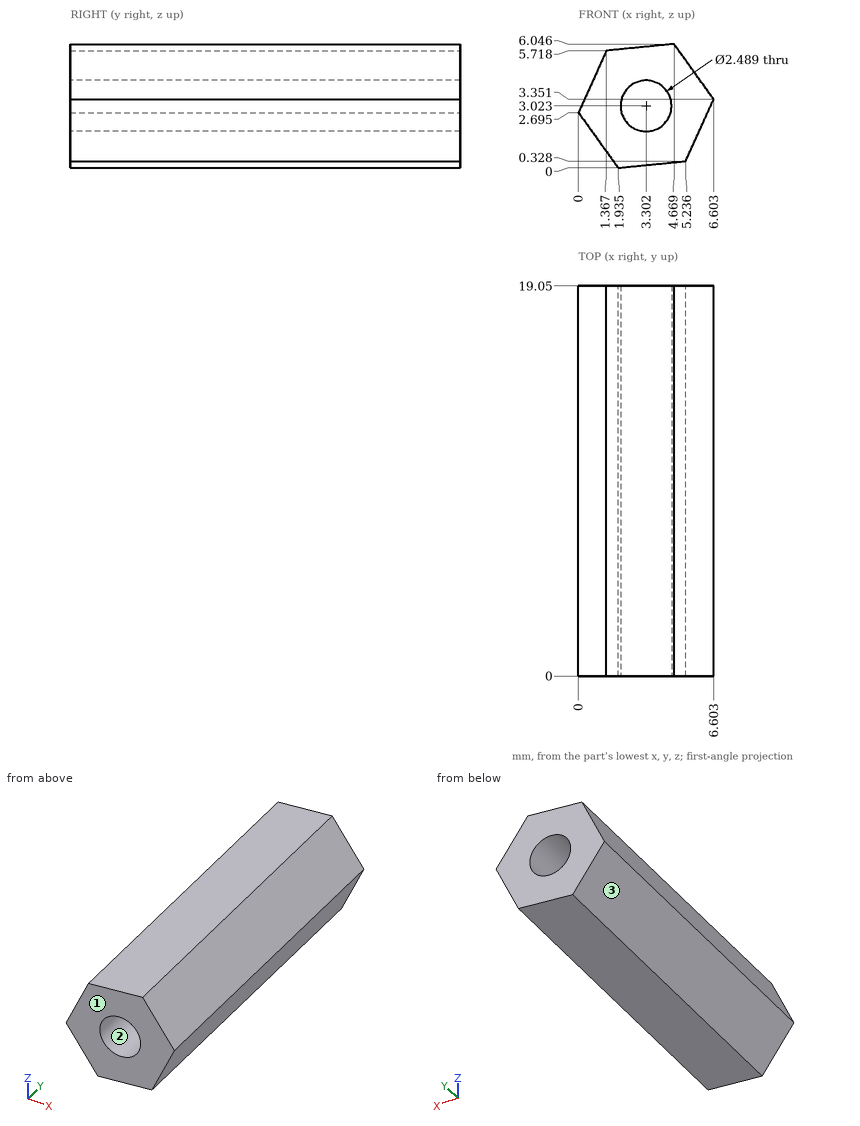
Here's the drawing with two shaded views (mm, measured from the low corner). I have some questions. Coordinates: 2 decimals unless noted, no trailing zeros. Answer in a Markdown table with one row per item.
(1) Will these pins go through, and if not, where does the flat tip stop? pin 1 Ø1.5 at (y, z) = (7, 3) entering from +X; pin 2 Ø3 at (y, z) = (12.5, 4.5) entering from -X.
Results found:
| item | result |
|---|---|
| pin 1 | stops at x = 6.6 |
| pin 2 | stops at x = 0.14 |
(2) If I drill on probe 1 along X at (y, z) = (13.25, 2) (1 decimal); probe 2 along Z at (x, y) = (2.5, 15.5) (1 decimal); probe 3 along X at (y, z) = (9.5, 2.25) (1 decimal), over which ranges is the centre line in solid material (lowest first)?
Results found:
| item | result |
|---|---|
| probe 1 | x = 0.5 to 2.6, 4 to 6 |
| probe 2 | z = 0.1 to 2.1, 4 to 5.8 |
| probe 3 | x = 0.3 to 2.3, 4.3 to 6.1 |
(3) Thinking about a two-plate mould opening in Z: for the marked faces 1, 2 and 3, which applies, released by +Z, released by -Z, zero draft, split by the parting line, or undercut?
Results found:
| item | result |
|---|---|
| face 1 | zero draft |
| face 2 | undercut |
| face 3 | released by -Z |
